Part print with two shaded views. Sizes in mm from the minimum x, y, z corner. A direction names the side the tool comes from. Coordinates: 2 decimals unless noted, no trailing zeros. Write each loop counter-clockwise with the first axis right and the second up, starting at its lowest first coordinate (ties: lowest second). Pieces come first, ordered by that corner, then holes.
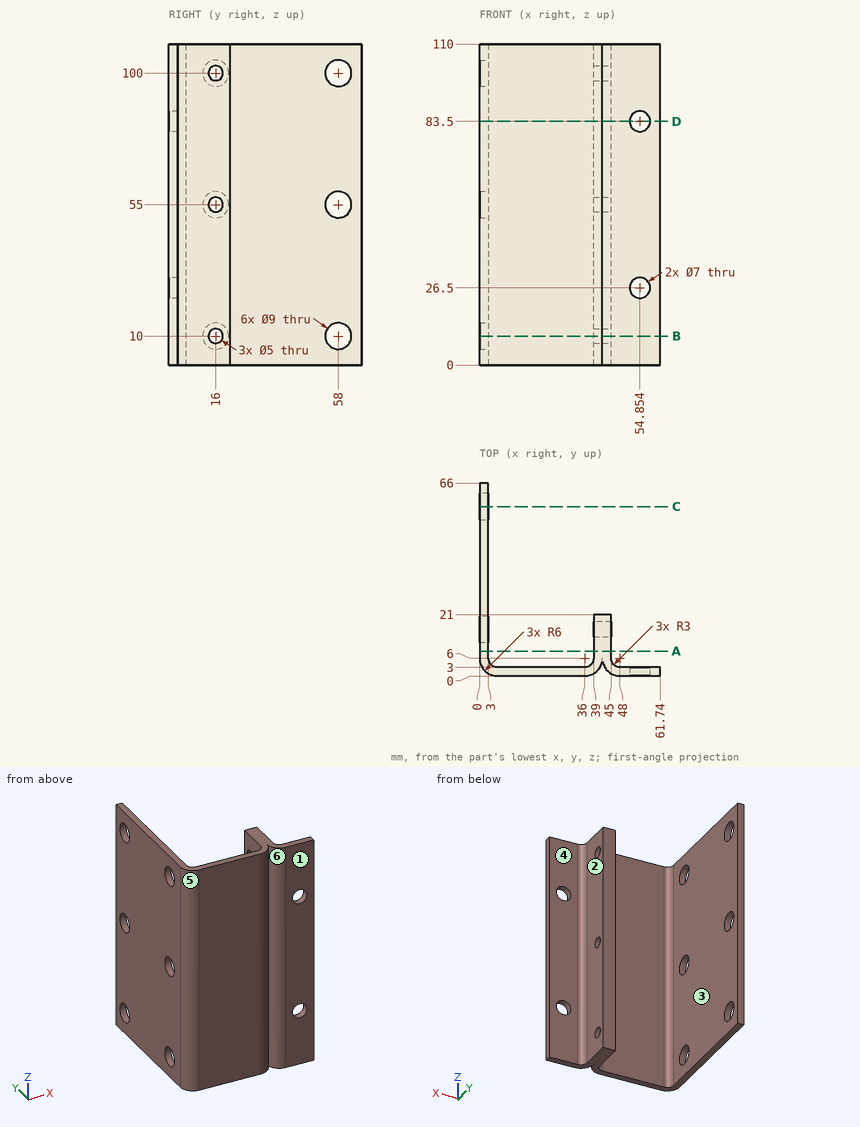
(1) 3-axis set-ups, long thin cutter, end or side, ignore diameter. For the marked faces 1, 2 and 3: which of +Z, -Z, +X, -X, +Y, -Y reach the whole face in a straight line?
(2) Flat gauge pins, fed straight in: P1, Ø1.8, axis at x = 41, z = 56, coming from the +Y side; P2, Ø1.5, axis at y = 10.5, z = 82, coming from the +X side; P3, Ø8, axis at y = 16, z = 100, coming from the -X side. Where does each tip first touch, or does it go through?
(3) Slice it at C-C, the plane y = 58. List the corners of the cut face in (x, z).
(4) Slice it at D-D, the plane z = 83.5. List the corners of the cut face in (x, y).
(5) Two-plate mould, pull along X, no slides. Class the marked faces 4, 5 and 6: pulls with the +X half, pulls with the -X half, needs draft (parallel to the pull), parting line crosses it, or undercut.
(6) Slice it at A-A, the plane y = 8.5. List the corners of the cut face in (x, z).
(7) Slice it at B-B, the plane z = 10. Give the number of separate pieces and of enclosed holes in the cut face, and give its area (3 significant figures).
(8) Probe L1, parallel to Z at x = 1.9, y = 16; L2, parallel to X at y = 15, z = 38; L3, parallel to X at y = 1, z = 83 (1 decimal). List the from-to ranges inside material, lowest first.
Results:
1. face 1: +Z, -Z, +X, -X, -Y
1. face 2: +Z, -Z, +X, +Y
1. face 3: +Z, -Z, +Y
2. P1: stops at y = 21
2. P2: stops at x = 45
2. P3: stops at x = 39
3. outline: (0, 0) - (3, 0) - (3, 5.5) - (0, 5.5) - close; (0, 14.5) - (3, 14.5) - (3, 50.5) - (0, 50.5) - close; (0, 59.5) - (3, 59.5) - (3, 95.5) - (0, 95.5) - close; (0, 104.5) - (3, 104.5) - (3, 110) - (0, 110) - close
4. outline: (0, 6) arc R6 ccw to (6, 0) - (36, 0) arc R6 ccw to (42, 6) arc R6 ccw to (48, 0) - (51.35, 0) - (51.35, 3) - (48, 3) arc R3 cw to (45, 6) - (45, 21) - (39, 21) - (39, 6) arc R3 cw to (36, 3) - (6, 3) arc R3 cw to (3, 6) - (3, 66) - (0, 66) - close; (58.35, 0) - (61.74, 0) - (61.74, 3) - (58.35, 3) - close
5. face 4: needs draft
5. face 5: pulls with the -X half
5. face 6: undercut
6. outline: (0, 0) - (3, 0) - (3, 110) - (0, 110) - close; (39, 0) - (45, 0) - (45, 110) - (39, 110) - close
7. separate pieces: 4
7. enclosed holes: 0
7. area: 381 mm2
8. L1: z = 0 to 5.5, 14.5 to 50.5, 59.5 to 95.5, 104.5 to 110
8. L2: x = 0 to 3, 39 to 45
8. L3: x = 2.7 to 39.3, 44.7 to 51.4, 58.3 to 61.7
